from build123d import *

# Parameters (mm, degrees)
SKETCH1_R           = 5.08
BOSS_EXTRUDE1_DEPTH = 15.24
SKETCH2_R           = 6.6675
BOSS_EXTRUDE2_DEPTH = 101.6
FILLET1_R           = 2.54


with BuildPart() as part:
    # Sketch1 → Boss-Extrude1 (new body)
    with BuildSketch(Plane.XY):
        Circle(SKETCH1_R)
    extrude(amount=-BOSS_EXTRUDE1_DEPTH)

    # Sketch2 → Boss-Extrude2 (add)
    with BuildSketch(Plane.XY):
        with Locations(Location((0, 0, 0), (0, 0, 180))):
            Circle(SKETCH2_R)
    extrude(amount=BOSS_EXTRUDE2_DEPTH)

    # Fillet1
    fillet1_edges = [part.edges().sort_by_distance(p)[0] for p in [
        (6.6675, 0, 101.6),
    ]]
    fillet(fillet1_edges, radius=FILLET1_R)


solid = part.part
Geometry check sheet. Reference: the model listing, model coordinates, mm. A direction names the side the tool comes from. Give positions to 0.01 mm unless a question says otherwise; leave off trailing zeros. Order: outer loops, then holes, each group sorted by start corner. A loop starts at its lowest first (then second) coordinate and runs counter-clockwise, first axis right, second up.
1) Cross-section at A-A (y = 0). Record the boundary of the cut face in (x, z), then the cut area to 3 significant figures.
Results are:
outline: (-6.67, 0) - (-5.08, 0) - (-5.08, -15.24) - (5.08, -15.24) - (5.08, 0) - (6.67, 0) - (6.67, 99.06) arc R2.54 ccw to (4.13, 101.6) - (-4.13, 101.6) arc R2.54 ccw to (-6.67, 99.06) - close
area: 1,510 mm2
2) Material ranges on probe 1 along Y at (x, z) = (0.5, 17); probe 2 along Y at (x, z) = (1, -7); probe 3 along X at (y, z) = (2.75, 87), recorded low to high.
Results are:
probe 1: y = -6.65 to 6.65
probe 2: y = -4.98 to 4.98
probe 3: x = -6.07 to 6.07
3) Gauge pin test, flat ends, axial feed: pin 1 (1.5 mm diameter, centred on x = -3, z = 30.5, fed in from -Y); pin 2 (1.5 mm diameter, centred on y = 4, z = 86.5, fed in from +X). Record the tip position at first contact, or that the pin passes through.
Results are:
pin 1: stops at y = -6.28
pin 2: stops at x = 5.82
4) Cross-section at C-C (z = -8). Record the boundary of the cut face in (x, y), then the cut area to 3 significant figures.
Results are:
outline: circle Ø10.16 at (0, 0)
area: 81.1 mm2
5) Cross-section at D-D (z = 91). Record the boundary of the cut face in (x, y) (1 decimal).
Results are:
outline: circle Ø13.3 at (0, 0)
6) Tool access check on faces 1 (the flat face through (2, 5, 0)), 2 (the flat face through (0, 0, -15.24)). Record the directions out of +Z, -Z, +X, -X, +Y, -Y that give a thin tool (end or side, any length) a straight path to the whole face; none if there is none.
Results are:
face 1: -Z
face 2: -Z, +X, -X, +Y, -Y
